Verification items for the finished model (mm, model axes). Round coordinates to 2 decimals unless told otherwise and drop trailing zeros. Order: outer loops, then holes, each group sorted by start corner. A loop starts at its lowest first (then second) coordinate and runs counter-clockwise, first axis right, second up. Notation, with made-up numbers: M 1.25,0.5 L 14.25,0.5 A16 cw 14.25,4.5 Z; hole C -3,6.25 d3. An arc over 180 degrees is marked long. One line per item, written item: value. Start each with the question number.
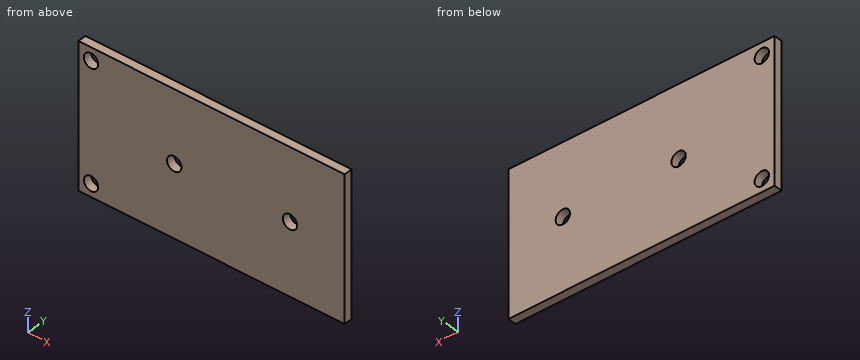
from build123d import *

# Parameters (mm, degrees)
SKETCH1_W            = 65
SKETCH1_H            = 33.5
BOSS_EXTRUDE1_DEPTH  = 2
M3_CLEARANCE_HOLE1_D = 3.4
M3_CLEARANCE_HOLE2_D = 3.4
SKETCH6_W            = 2
SKETCH6_H            = 33.5
CUT_EXTRUDE1_DEPTH   = 3


with BuildPart() as part:
    # Sketch1 → Boss-Extrude1 (new body)
    with BuildSketch(Plane(origin=(0, 0, 0), x_dir=(1, 0, 0), z_dir=(0, 1, 0))):
        with Locations((-39.686085356, 13.7444519)):
            Rectangle(SKETCH1_W, SKETCH1_H)
    extrude(amount=BOSS_EXTRUDE1_DEPTH)

    # M3 Clearance Hole1 (through all)
    with Locations(Plane(origin=(0, 2, 0), x_dir=(1, 0, 0), z_dir=(0, 1, 0))):
        with Locations((-67.186085356, 27.4944519), (-67.186085356, -0.0055481)):
            Hole(M3_CLEARANCE_HOLE1_D / 2)

    # M3 Clearance Hole2 (through all)
    with Locations(Plane(origin=(-47.486085356, 2, -13.7444519), x_dir=(0, 0, 1), z_dir=(0, 1, 0))):
        with Locations((0, 0), (0, 27.4)):
            Hole(M3_CLEARANCE_HOLE2_D / 2)

    # Sketch6 → Cut-Extrude1 (cut, through all)
    with BuildSketch(Plane.XZ):
        with Locations((-71.186085356, -13.7444519)):
            Rectangle(SKETCH6_W, SKETCH6_H)
    extrude(amount=-CUT_EXTRUDE1_DEPTH, mode=Mode.SUBTRACT)


solid = part.part
1. Section check B-B (y = 1.05). Record the cut outline in (x, z), and give its area (3 significant figures).
2. Depth check by flat-ended pin: pin 1 (3 mm diameter, centred on x = -67.19, z = -27.49, fed in from +Y); pin 2 (4.5 mm diameter, centred on x = -67.19, z = 0.01, fed in from -Y). Enter the tip coordinate at first touch or a pass-through.
3. Scan lines: line 1 along Z through (x, y) = (-47.5, 1.75); line 2 along X through (y, z) = (1.3, -13.5); line 3 along X through (y, z) = (0.5, -1.5). Record each from-to range of solid material in increasing order.
4. Section check A-A (z = -13.5). Record the cut outline in (x, y), and give its area (3 significant figures).
Geometry check:
1. outline: M -70.19,-30.49 L -7.19,-30.49 L -7.19,3.01 L -70.19,3.01 Z; hole C -67.19,-27.49 d3.4; hole C -67.19,0.01 d3.4; hole C -47.49,-13.74 d3.4; hole C -20.09,-13.74 d3.4
1. area: 2,070 mm²
2. pin 1: passes through
2. pin 2: stops at y = 0
3. line 1: z = -30.49 to -15.44, -12.04 to 3.01
3. line 2: x = -70.19 to -49.17, -45.8 to -21.77, -18.4 to -7.19
3. line 3: x = -70.19 to -67.98, -66.4 to -7.19
4. outline: M -70.19,0 L -49.17,0 L -49.17,2 L -70.19,2 Z; M -45.8,0 L -21.77,0 L -21.77,2 L -45.8,2 Z; M -18.4,0 L -7.19,0 L -7.19,2 L -18.4,2 Z
4. area: 113 mm²
